Print and shaded views of the part. All mm, measured from the part's lowest x, y and z. A direction names the side the tool comes from. Round coordinates to 2 decimals unless told otherwise and drop trailing zeros. Loops run counter-clockwise (first coordinate to the right, second up) from the corner with the lowest first, then second, coordinate; pieces in that order, holes last. Notation, with made-up numbers: (-33.5, 34) -> (3.5, 34) arc R23 ccw to (3.5, 48) -> close; hole circle Ø3 at (11.25, -27). An arc over 180 degrees is marked (long way). Use a Markdown table: item, result.
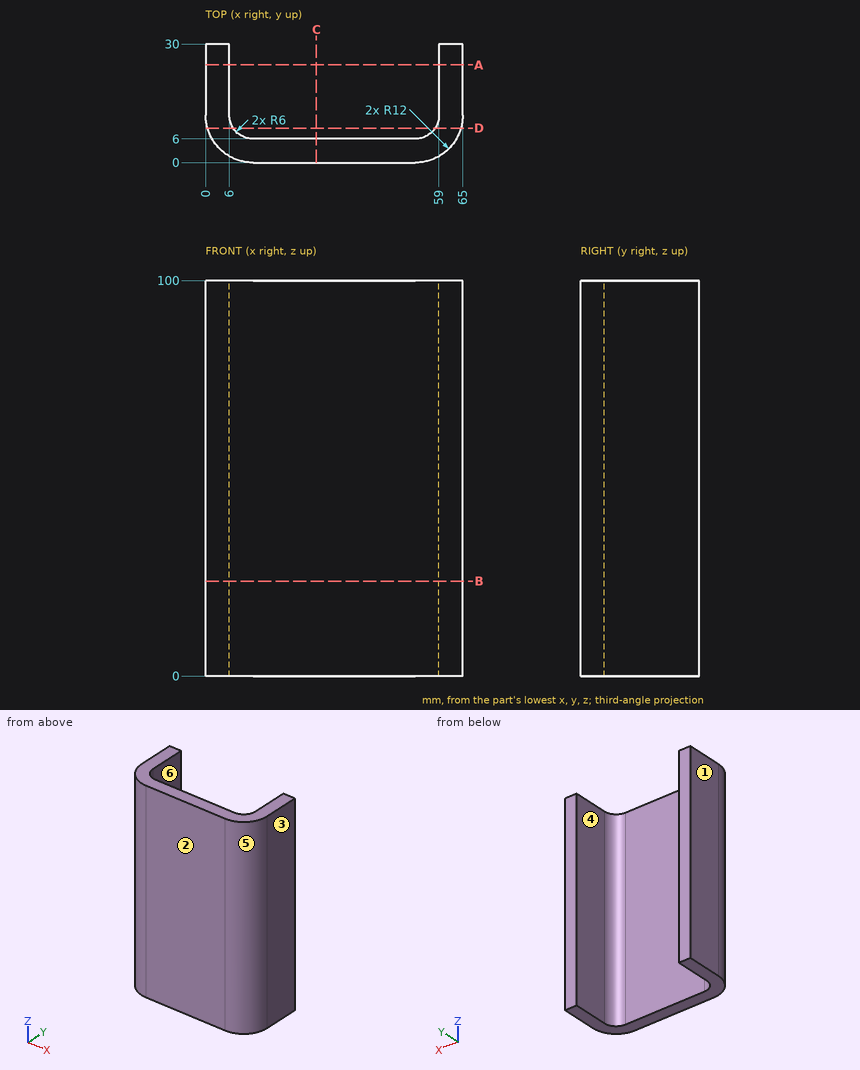
Q1. Band-saw the part on A-A, the plane y = 24.75. Give the cut face in (x, z).
Results list:
| item | result |
|---|---|
| outline | (0, 0) -> (6, 0) -> (6, 100) -> (0, 100) -> close; (59, 0) -> (65, 0) -> (65, 100) -> (59, 100) -> close |
Q2. Band-saw the part on C-C, the plane x = 28. Give the cut face in (y, z), plus the area to 3 significant figures.
Results list:
| item | result |
|---|---|
| outline | (0, 0) -> (6, 0) -> (6, 100) -> (0, 100) -> close |
| area | 600 mm² |
Q3. Flat gauge pins, fed straight in: pin 1 (6 mm diameter, centred on x = 30, z = 41, fed in from +Y); pin 2 (1 mm diameter, centred on y = 5.5, z = 11.5, fed in from +X); pin 3 (4 mm diameter, centred on x = 10.5, z = 76, fed in from +Y). Where does each tip first touch, or does it go through?
Results list:
| item | result |
|---|---|
| pin 1 | stops at y = 6 |
| pin 2 | stops at x = 63.39 |
| pin 3 | stops at y = 7.13 |
Q4. Pull direction X, two halves, no side cores. Call the marked faces 1, 2, 3 and 4: released by +X, released by -X, zero draft, split by the parting line, or undercut.
Results list:
| item | result |
|---|---|
| face 1 | released by -X |
| face 2 | zero draft |
| face 3 | released by +X |
| face 4 | undercut |
Q5. Band-saw the part on B-B, the plane z = 24. Give the cut face in (x, y).
Results list:
| item | result |
|---|---|
| outline | (0, 12) arc R12 ccw to (12, 0) -> (53, 0) arc R12 ccw to (65, 12) -> (65, 30) -> (59, 30) -> (59, 12) arc R6 cw to (53, 6) -> (12, 6) arc R6 cw to (6, 12) -> (6, 30) -> (0, 30) -> close |
Q6. Band-saw the part on D-D, the plane y = 8.75. Give the cut face in (x, z), plus the area to 3 significant figures.
Results list:
| item | result |
|---|---|
| outline | (0.45, 0) -> (6.96, 0) -> (6.96, 100) -> (0.45, 100) -> close; (58.04, 0) -> (64.55, 0) -> (64.55, 100) -> (58.04, 100) -> close |
| area | 1,300 mm² |
Q7. Drill centre lines: L1, parallel to X at y = 15, z = 65.5; L2, parallel to Y at x = 14, z = 83.5; L3, parallel to X at y = 10, z = 85. Where is each one in solid material? Low to high. Write a range as from..to.
Results list:
| item | result |
|---|---|
| L1 | x = 0..6, 59..65 |
| L2 | y = 0..6 |
| L3 | x = 0.17..6.34, 58.66..64.83 |
Q8. Tool access for the marked faces 5 and 6: list every direction of +Z, -Z, +X, -X, +Y, -Y with a clear straight run to the whole face (end or side of a thin tool).
Results list:
| item | result |
|---|---|
| face 5 | +Z, -Z, +X, -Y |
| face 6 | +Z, -Z, +Y |
